Here's the drawing with two shaded views (mm, measured from the low corner). I have some questions. A direction names the side the tool comes from. Coordinates: 2 decimals unless noted, no trailing zeros. Write each loop counter-clockwise with the first axis right and the second up, starting at its lowest first coordinate (ties: lowest second). Pieces come first, ordered by that corner, then holes.
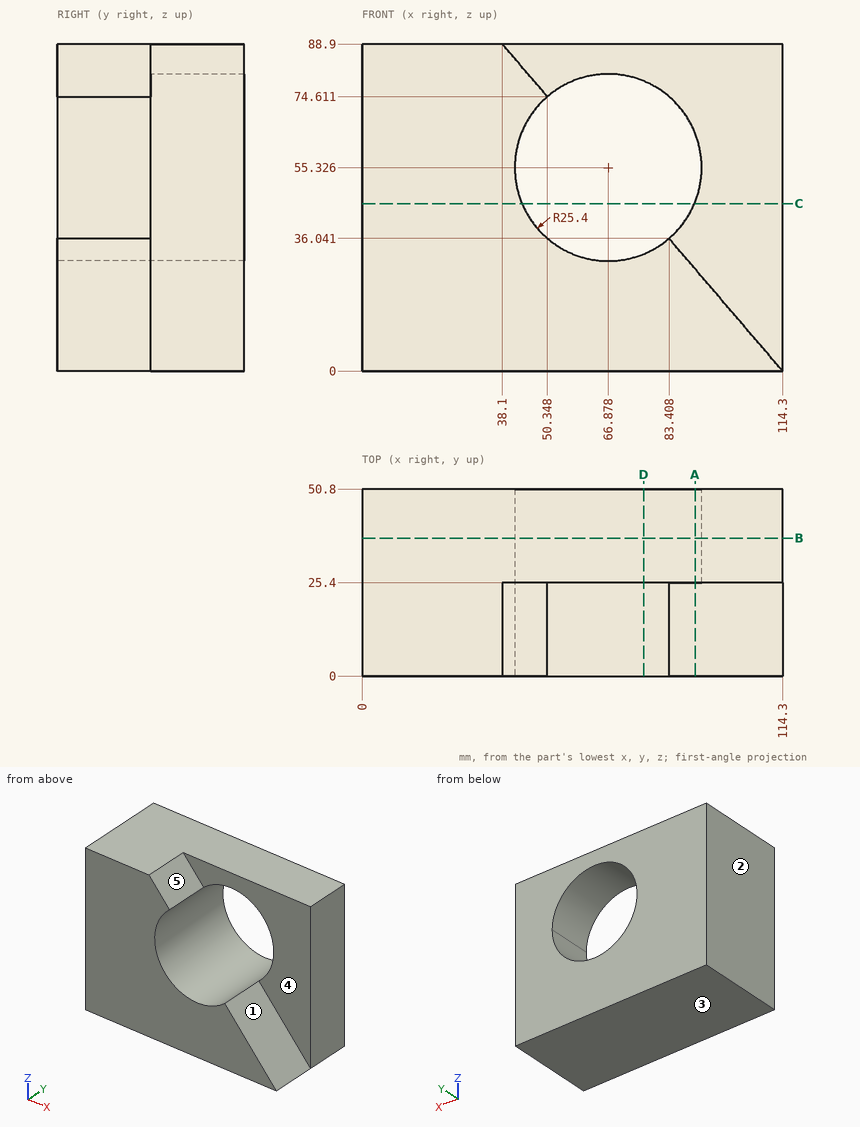
1. If we mould it in two halves opening along Z, with no side actions, what happens to the marked faces 3, 4 and 5? For each: pulls with the +Z half, pulls with the -Z half, needs draft (parallel to the pull), parting line crosses it, or undercut.
Verdict:
face 3: pulls with the -Z half
face 4: needs draft
face 5: pulls with the +Z half
2. Please list where these lines run through material, in increasing order: line 1 along Y through (x, z) = (95, 40.5); line 2 along X through (y, z) = (41, 67.5) (1 decimal); line 3 along X through (y, z) = (37, 70) (1 decimal).
Verdict:
line 1: y = 25.4 to 50.8
line 2: x = 0 to 44.6, 89.2 to 114.3
line 3: x = 0 to 46.1, 87.6 to 114.3
3. I want a section at C-C on z = 45.5. Please give me the cut outline in (x, y) (1 decimal), plus the area to 3 significant figures.
Verdict:
outline: (0, 0) - (43.5, 0) - (43.5, 50.8) - (0, 50.8) - close; (90.3, 25.4) - (114.3, 25.4) - (114.3, 50.8) - (90.3, 50.8) - close
area: 2,820 mm2
4. I want a section at B-B on y = 37.5. Please give me the cut outline in (x, z).
Verdict:
outline: (0, 0) - (114.3, 0) - (114.3, 88.9) - (0, 88.9) - close; hole circle Ø50.8 at (66.88, 55.33)
5. On a 3-axis mill with a long thin cutter (end or side, diameter ignored), from which of +Z, -Z, +X, -X, +Y, -Y can I reach the whole of each face in a straight line? I mean the marked faces 1 and 2. Say none if no direction works.
Verdict:
face 1: +Z, +X, -Y
face 2: +Z, -Z, -X, +Y, -Y
6. I want a section at D-D on x = 76.5. Please give me the cut outline in (y, z).
Verdict:
outline: (0, 0) - (50.8, 0) - (50.8, 31.82) - (0, 31.82) - close; (25.4, 78.83) - (50.8, 78.83) - (50.8, 88.9) - (25.4, 88.9) - close
7. I want a section at A-A on x = 90.5. Please give me the cut outline in (y, z), plus the area to 3 significant figures.
Verdict:
outline: (0, 0) - (50.8, 0) - (50.8, 45.99) - (25.4, 45.99) - (25.4, 27.77) - (0, 27.77) - close; (25.4, 64.66) - (50.8, 64.66) - (50.8, 88.9) - (25.4, 88.9) - close
area: 2,490 mm2
8. For pin 1 (3 mm diameter, centred on x = 101.5, z = 65, fed in from -Y); pin 2 (1 mm diameter, centred on y = 23.5, z = 68.5, fed in from +X), each with a flat end and sliding along its axis, tell me the tip position at first contact or that it passes through.
Verdict:
pin 1: stops at y = 25.4
pin 2: stops at x = 45.47
